Build history of the part. All positions in model axes, mm. Face numbers are marked on the shaded views. A direction names the side the tool comes from. Coordinates: 2 decimals unless noted, no trailing zeros. Write each loop counter-clockwise with the first axis right and the second up, starting at its lowest first coordinate (ties: lowest second). Pieces come first, ordered by that corner, then holes.
```python
from build123d import *

# Parameters (mm, degrees)
EXTRUDE_1_DEPTH        = 4
SKETCH_3_W             = 10
SKETCH_3_H             = 2.5
EXTRUDE_2_DEPTH        = 4
FILLET_1_R             = 3
HOLE_WIZARD_M8_1_D     = 6.8
HOLE_WIZARD_M8_1_DEPTH = 19.75
HOLE_WIZARD_M8_1_TIP   = 2.042926105


with BuildPart() as part:
    # 草图1 → 凸台-拉伸1 (new, symmetric)
    with BuildSketch(Plane.XY):
        with BuildLine():
            Line((16.832132438, -5), (2.667867562, -5))
            ThreePointArc((2.667867562, -5), (0.969162586, -3.499129927), (0, -1.45))
            Line((0, -1.45), (0, 0))
            Line((0, 0), (19.5, 0))
            Line((19.5, 0), (19.5, -1.45))
            ThreePointArc((19.5, -1.45), (18.530837414, -3.499129927), (16.832132438, -5))
        make_face()
    extrude(amount=EXTRUDE_1_DEPTH, both=True)

    # 草图3 → 凸台-拉伸2 (add, symmetric)
    with BuildSketch(Plane.XY):
        with Locations((9.75, 1.25)):
            Rectangle(SKETCH_3_W, SKETCH_3_H)
    extrude(amount=EXTRUDE_2_DEPTH, both=True)

    # 圆角1
    fillet_1_edges = [part.edges().sort_by_distance(p)[0] for p in [
        (19.5, -0.725, 4),
        (0, -0.725, -4),
        (4.75, 1.25, -4),
        (14.75, 1.25, 4),
    ]]
    fillet(fillet_1_edges, radius=FILLET_1_R)

    # M8 螺纹孔1
    with Locations(Plane(origin=(9.75, 2.5, 0), x_dir=(0, 0, 1), z_dir=(0, 1, 0))):
        with Locations((0, 0)):
            Hole(HOLE_WIZARD_M8_1_D / 2, depth=HOLE_WIZARD_M8_1_DEPTH)
            with Locations((0, 0, -(HOLE_WIZARD_M8_1_DEPTH + HOLE_WIZARD_M8_1_TIP / 2))):  # 118° drill point
                Cone(0, HOLE_WIZARD_M8_1_D / 2, HOLE_WIZARD_M8_1_TIP, mode=Mode.SUBTRACT)


solid = part.part
```
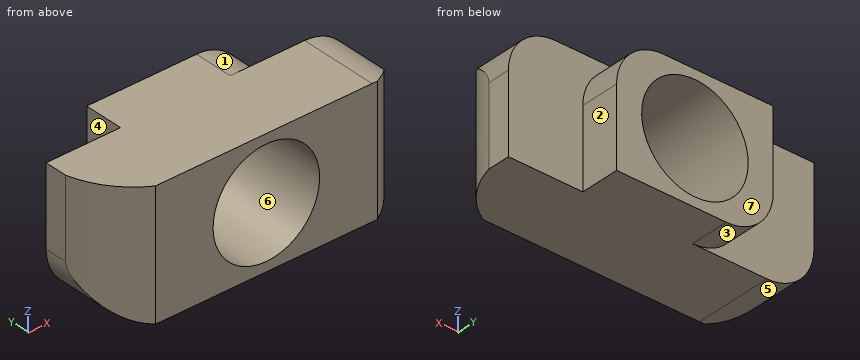
1. Flat gauge pins, fed straight in: pin 1 (1.5 mm diameter, centred on y = -2, z = -3, fed in from -X); pin 2 (0.8 mm diameter, centred on y = 2, z = -1, fed in from +X); pin 3 (1 mm diameter, centred on x = 4, z = 3, fed in from +Y); pin 4 (2.5 mm diameter, centred on x = 15, z = -1.5, fed in from +Y). Where does each tip first touch, or does it go through?
Computed values:
pin 1: stops at x = 0.27
pin 2: stops at x = 14.75
pin 3: stops at y = 0
pin 4: stops at y = 2.5
2. Saw through at C-C on y = -0.5. List the corners of the cut face in (x, z).
Computed values:
outline: (0, -1) arc R3 ccw to (3, -4) - (19.5, -4) - (19.5, 1) arc R3 ccw to (16.5, 4) - (0, 4) - close; hole circle Ø6.8 at (9.75, 0)
3. Saw through at B-B on x = 9.75. List the corners of the cut face in (y, z).
Computed values:
outline: (-5, -4) - (2.5, -4) - (2.5, -3.4) - (-5, -3.4) - close; (-5, 3.4) - (2.5, 3.4) - (2.5, 4) - (-5, 4) - close
4. Probe line 1 along X through (y, z) = (-1.25, -1); line 2 along X through (y, z) = (-3, -0.25); line 3 along Z through (x, y) = (8.5, -2). List the from-to ranges inside material, lowest first.
Computed values:
line 1: x = 0 to 6.5, 13 to 19.5
line 2: x = 0.63 to 6.36, 13.14 to 18.87
line 3: z = -4 to -3.16, 3.16 to 4
5. 3-axis set-ups, long thin cutter, end or side, ignore diameter. For the marked faces 1, 2, 3 and 4: which of +Z, -Z, +X, -X, +Y, -Y reach the whole face in a straight line?
Computed values:
face 1: +Z, +X, +Y
face 2: +Z, -Z, +X, +Y
face 3: -Z, -X, +Y
face 4: +Z, -Z, -X, +Y
6. Saw through at A-A on z = 0. List the corners of the cut face in (x, y).
Computed values:
outline: (0, -1.45) arc R5.63 ccw to (2.67, -5) - (6.35, -5) - (6.35, 2.5) - (4.75, 2.5) - (4.75, 0) - (0, 0) - close; (13.15, -5) - (16.83, -5) arc R5.63 ccw to (19.5, -1.45) - (19.5, 0) - (14.75, 0) - (14.75, 2.5) - (13.15, 2.5) - close
7. Mould opens along X. For the marked faces 5, 6 and 7 say: +X half, -X half, draft (parallel to the pull), parting line (faces both ways), or undercut.
Computed values:
face 5: -X half
face 6: undercut
face 7: draft
8. Saw through at D-D on z = -2.5. List the corners of the cut face in (x, y).
Computed values:
outline: (0.4, -2.57) arc R5.63 ccw to (2.67, -5) - (7.45, -5) - (7.45, 2.5) - (5.15, 2.5) - (5.15, 0) - (0.4, 0) - close; (12.05, -5) - (16.83, -5) arc R5.63 ccw to (19.5, -1.45) - (19.5, 0) - (14.75, 0) - (14.75, 2.5) - (12.05, 2.5) - close
